```python
from build123d import *

# Parameters (mm, degrees)
F1_W      = 12.5
F1_H      = 5.75
F2_DEPTH  = 7
F3_W      = 11.7
F3_H      = 4.95
F4_DEPTH  = 6.4
F5_W      = 0.64
F5_H      = 0.64
F6_DEPTH  = 0.601
F7_W      = 0.9
F7_H      = 0.4
F8_DEPTH  = 4
F9_W      = 0.4
F9_H      = 1
F10_DEPTH = 4


# Not quite as in the source:
# - a feature names something its author has since deleted; it is built from what else it names


with BuildPart() as f2:
    # F1 (on Top) → F2 (new body)
    with BuildSketch(Plane.XY):
        with Locations((0, 0.32)):
            Rectangle(F1_W, F1_H)
    extrude(amount=F2_DEPTH)

    # F3 (on face) → F4 (cut)
    with BuildSketch(Plane.XY.offset(7)):
        with Locations((0, 0.32)):
            Rectangle(F3_W, F3_H)
    extrude(amount=-F4_DEPTH, mode=Mode.SUBTRACT)

    # F5 (on face) → F6 (cut, through all)
    with BuildSketch(Plane.XY.offset(0.6)):
        with Locations((-1.25, 0)):
            Rectangle(F5_W, F5_H)
        with Locations((-3.75, 0)):
            Rectangle(F5_W, F5_H)
        with Locations((1.25, 0)):
            Rectangle(F5_W, F5_H)
        with Locations((3.75, 0)):
            Rectangle(F5_W, F5_H)
    extrude(amount=-F6_DEPTH, mode=Mode.SUBTRACT)

    # F7 (on face) → F8 (cut)
    with BuildSketch(Plane.XY.offset(7)):
        with Locations((-4.95, -2.355)):
            Rectangle(F7_W, F7_H)
        with Locations((4.95, -2.355)):
            Rectangle(F7_W, F7_H)
    extrude(amount=-F8_DEPTH, mode=Mode.SUBTRACT)

    # F9 (on face) → F10 (cut)
    with BuildSketch(Plane.XY.offset(7)):
        with Locations((-6.05, 1.3)):
            Rectangle(F9_W, F9_H)
        with Locations((6.05, 1.3)):
            Rectangle(F9_W, F9_H)
    extrude(amount=-F10_DEPTH, mode=Mode.SUBTRACT)


solid = f2.part
```
Check sheet for the modelled part. Datum: model origin and axes. Units: mm. A direction names the side the tool comes from. Coordinates: 2 decimals unless noted, no trailing zeros. Loops run counter-clockwise (first coordinate to the right, second up) from the corner with the lowest first, then second, coordinate; pieces in that order, holes last. Notation, with made-up numbers: M -2,84 L 37,84 A21 ccw 37,112 Z; hole C 86.5,78.5 d3. An arc over 180 degrees is marked long. Answer as a JSON object with one key per item and string values.
1. Depth check by flat-ended pin: P1, Ø1.5, axis at x = -4, y = -0.5, coming from the +Z side. Enter the tip coordinate at first touch or a pass-through.
Outcome:
{"P1": "z = 0.6"}
2. Sectioned sample at C-C on y = 0.1. Record the cut outline in (x, z), and give its area (3 significant figures).
Outcome:
{"outline": "M -6.25,0 L -4.07,0 L -4.07,0.6 L -5.85,0.6 L -5.85,7 L -6.25,7 Z; M -3.43,0 L -1.57,0 L -1.57,0.6 L -3.43,0.6 Z; M -0.93,0 L 0.93,0 L 0.93,0.6 L -0.93,0.6 Z; M 1.57,0 L 3.43,0 L 3.43,0.6 L 1.57,0.6 Z; M 4.07,0 L 6.25,0 L 6.25,7 L 5.85,7 L 5.85,0.6 L 4.07,0.6 Z", "area": "11.1 mm²"}
3. Scan lines: L1, parallel to X at y = -1.9, z = 5.5; L2, parallel to Y at x = 3, z = 4 (3 decimals); L3, parallel to Z at x = -3, y = -1.85. Record each from-to range of solid material in increasing order. Write a range as from..to.
Outcome:
{"L1": "-6.25..-5.85, 5.85..6.25", "L2": "-2.555..-2.155, 2.795..3.195", "L3": "0..0.6"}
4. Sectioned sample at A-A on z = 5. Record the cut outline in (x, y) (3 decimals).
Outcome:
{"outline": "M -6.25,-2.555 L -5.4,-2.555 L -5.4,-2.155 L -5.85,-2.155 L -5.85,0.8 L -6.25,0.8 Z; M -6.25,1.8 L -5.85,1.8 L -5.85,2.795 L 5.85,2.795 L 5.85,1.8 L 6.25,1.8 L 6.25,3.195 L -6.25,3.195 Z; M -4.5,-2.555 L 4.5,-2.555 L 4.5,-2.155 L -4.5,-2.155 Z; M 5.4,-2.555 L 6.25,-2.555 L 6.25,0.8 L 5.85,0.8 L 5.85,-2.155 L 5.4,-2.155 Z"}
5. Access from +Z, -Z, +X, -X, +Y, -Y to the whole of each face (thin tool, end or side, straight path). Record for faces 4 (the flat face through (-5.85, 0, 4)), 5 (the flat face through (-6.25, 0, 3)).
Outcome:
{"face 4": "+Z", "face 5": "+Z, -Z, -X, +Y, -Y"}
6. Sectioned sample at B-B on z = 0.75. Record the cut outline in (x, y) (3 decimals), and give its area (3 significant figures).
Outcome:
{"outline": "M -6.25,-2.555 L 6.25,-2.555 L 6.25,3.195 L -6.25,3.195 Z; hole M -5.85,-2.155 L 5.85,-2.155 L 5.85,2.795 L -5.85,2.795 Z", "area": "14.0 mm²"}
7. Sectioned sample at D-D on x = -3.25. Record the cut outline in (y, z) (3 decimals).
Outcome:
{"outline": "M -2.555,0 L 3.195,0 L 3.195,7 L 2.795,7 L 2.795,0.6 L -2.155,0.6 L -2.155,7 L -2.555,7 Z"}
8. Release check for a two-part mould opening along X. For faces 1 (the flat face through (6, -1, 7)), 2 (the flat face through (5.85, 0, 4)), 3 (the flat face through (6.25, 0, 3)) record: pulls with the +X half, pulls with the -X half, needs draft (parallel to the pull), parting line crosses it, or undercut.
Outcome:
{"face 1": "needs draft", "face 2": "undercut", "face 3": "pulls with the +X half"}
